The model under review builds one solid part; all positions refer to its coordinate system, in mm. Face numbers are marked on the shaded views. A direction names the side the tool comes from. Round coordinates to 2 decimals unless told otherwise and drop trailing zeros. Write each loop counter-clockwise with the first axis right and the second up, starting at its lowest first coordinate (ties: lowest second). Pieces come first, ordered by that corner, then holes. Notation, with made-up numbers: (54.5, 28) - (65.5, 28) arc R16 ccw to (65.5, 37) - close; hole circle Ø5 at (27.25, 4.5). An arc over 180 degrees is marked (long way). Use one line per item in the form item = value.
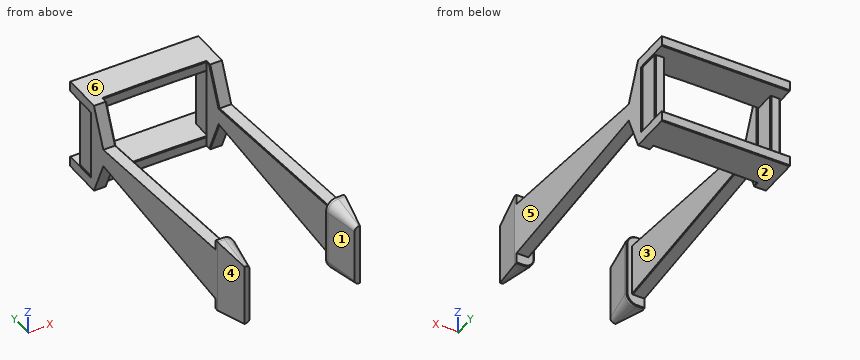
from build123d import *

# Parameters (mm, degrees)
BOSS_EXTRUDE1_DEPTH           = 30
SKETCH2_W                     = 26.926999998
SKETCH2_H                     = 60
BOSS_EXTRUDE2_DEPTH           = 200
BOSS_EXTRUDE3_START           = 30
BOSS_EXTRUDE3_DEPTH           = 30
BOSS_EXTRUDE4_DEPTH           = 4.0365
BOSS_EXTRUDE4_DEPTH_BACK      = 30.9635
BOSS_EXTRUDE5_DEPTH           = 10
FILLET1_R                     = 30
SKETCH7_W                     = 260
SKETCH7_H                     = 710
CUT_EXTRUDE1_DEPTH            = 768.843643003
CHAMFER1_SIZE                 = 2
CHAMFER2_SIZE                 = 2
CHAMFER3_SIZE                 = 2
CHAMFER4_SIZE                 = 2
CHAMFER6_SIZE                 = 2
BOSS_EXTRUDE6_DEPTH           = 99
BOSS_EXTRUDE6_DRAFT           = 10
BOSS_EXTRUDE6_PROFILE_2_DEPTH = 99
BOSS_EXTRUDE6_PROFILE_2_DRAFT = 10


with BuildPart() as part:
    # Sketch1 → Boss-Extrude1 (new body)
    with BuildSketch(Plane.XY):
        with BuildLine():
            Line((0, 0), (361.02, 0))
            Line((361.02, 0), (361.02, -100))
            Line((361.02, -100), (326.02, -100))
            ThreePointArc((326.02, -100), (180.51, -98.235310481), (35, -100))
            Line((35, -100), (0, -100))
            Line((0, -100), (0, 0))
        make_face()
    extrude(amount=BOSS_EXTRUDE1_DEPTH)

    # Sketch2 → Boss-Extrude2 (add)
    with BuildSketch(Plane(origin=(0, 0, 0), x_dir=(-1, 0, 0), z_dir=(0, 0, -1))):
        with Locations((-343.52, -70)):
            Rectangle(SKETCH2_W, SKETCH2_H)
        with Locations((-17.5, -70)):
            Rectangle(SKETCH2_W, SKETCH2_H)
    extrude(amount=BOSS_EXTRUDE2_DEPTH)

    # Sketch3 → Boss-Extrude3 (add)
    with BuildSketch(Plane(origin=(0, 0, -200), x_dir=(-1, 0, 0), z_dir=(0, 0, -1)).offset(BOSS_EXTRUDE3_START)):
        with BuildLine():
            Line((0, -100), (0, 0))
            Line((0, 0), (-361.02, 0))
            Line((-361.02, 0), (-361.02, -100))
            Line((-361.02, -100), (-326.02, -100))
            ThreePointArc((-326.02, -100), (-180.51, -98.235310481), (-35, -100))
            Line((-35, -100), (0, -100))
        make_face()
    extrude(amount=-BOSS_EXTRUDE3_DEPTH)

    # Sketch5 → Boss-Extrude4 (add, two sides: drawn at the far end of the back side and taken through both)
    with BuildSketch(Plane.ZY.offset(-4.036500001).offset(-BOSS_EXTRUDE4_DEPTH_BACK)):
        Polygon((-200, -100), (0, -100), (30, -100), (30, -115), (-75, -160), (-25, -700), (-100, -700), (-175, -700), (-125, -160), (-230, -115), (-230, -100), align=None)
    extrude(amount=BOSS_EXTRUDE4_DEPTH + BOSS_EXTRUDE4_DEPTH_BACK)

    # Sketch6 → Boss-Extrude5 (add)
    with BuildSketch(Plane.XZ.offset(700)):
        Polygon((0, -25), (0, 5), (50, 5), (50, -205), (0, -205), (0, -175), align=None)
    extrude(amount=BOSS_EXTRUDE5_DEPTH)

    # Fillet1
    fillet1_edges = [part.edges().sort_by_distance(p)[0] for p in [
        (50, -705, -205),
        (50, -705, 5),
    ]]
    fillet(fillet1_edges, radius=FILLET1_R)

    # Sketch7 → Cut-Extrude1 (cut, through all)
    with BuildSketch(Plane(origin=(180.51, 0, 0), x_dir=(0, 0, -1), z_dir=(1, 0, 0))):
        with Locations((100, -355)):
            Rectangle(SKETCH7_W, SKETCH7_H)
    extrude(amount=CUT_EXTRUDE1_DEPTH, mode=Mode.SUBTRACT)

    # Mirror2: part across plane


with BuildPart() as part_1:
    add(part.part)
    add(part.part.mirror(Plane(origin=(180.51, 0, 0), x_dir=(0, 0, 1), z_dir=(1, 0, 0))))

    # Chamfer1
    chamfer1_edges = [part_1.edges().sort_by_distance(p)[0] for p in [
        (180.51, 0, 30),
        (180.51, 0, 0),
        (180.51, 0, -200),
        (180.51, 0, -230),
    ]]
    chamfer(chamfer1_edges, length=CHAMFER1_SIZE)

    # Chamfer2
    chamfer2_edges = [part_1.edges().sort_by_distance(p)[0] for p in [
        (356.983499999, -40, -100),
        (330.056500001, -40, -100),
        (4.036500001, -40, -100),
        (30.963499999, -40, -100),
    ]]
    chamfer(chamfer2_edges, length=CHAMFER2_SIZE)

    # Chamfer3
    chamfer3_edges = [part_1.edges().sort_by_distance(p)[0] for p in [
        (326.019999999, -107.5, -230),
        (326.019999999, -137.5, -177.5),
        (326.019999999, -430, -150),
        (326.019999999, -430, -50),
        (326.019999999, -137.5, -22.5),
        (326.019999999, -107.5, 30),
        (35.000000001, -107.5, 30),
        (35.000000001, -137.5, -22.5),
        (35.000000001, -430, -50),
        (35.000000001, -430, -150),
        (35.000000001, -137.5, -177.5),
        (35.000000001, -107.5, -230),
    ]]
    chamfer(chamfer3_edges, length=CHAMFER3_SIZE)

    # Chamfer4
    chamfer4_edges = [part_1.edges().sort_by_distance(p)[0] for p in [
        (50, -700, -100),
        (10, -700, 5),
        (41.213203436, -700, -3.786796564),
        (41.213203436, -700, -196.213203436),
        (311.02, -700, -100),
        (351.02, -700, 5),
        (351.02, -700, -205),
        (319.806796564, -700, -196.213203436),
        (319.806796564, -700, -3.786796564),
        (10, -700, -205),
    ]]
    chamfer(chamfer4_edges, length=CHAMFER4_SIZE)

    # Chamfer6
    # the kernel refuses this chamfer: 2 mm, written as the material it takes off along each edge
    with BuildSketch(Plane(origin=(180.51, -6098.235310479, 30), x_dir=(0.025441959758898923, 0.9996763009512762, 0), z_dir=(0.9996763009512762, -0.025441959758898923, 0))) as chamfer6_piece_1_section:
        Polygon((5999.999999998 + CHAMFER6_SIZE, 0), (5999.999999998, -CHAMFER6_SIZE), (5999.999999998, 0), align=None)
    chamfer6_piece_1 = revolve(axis=Axis((180.51, -6098.235310479, 30), (0, 0, 1)), revolution_arc=2.915748449, mode=Mode.PRIVATE)
    chamfer6_piece_1 = split(chamfer6_piece_1, bisect_by=Plane(origin=(327.145000629, -99.268037673, 29.12500063), z_dir=(-0.7071067811865476, 0, 0.7071067811865476)), keep=Keep.TOP, mode=Mode.PRIVATE)
    chamfer6_piece_1 = split(chamfer6_piece_1, bisect_by=Plane(origin=(180.135000332, -99.268037673, -117.135000331), z_dir=(0.7071067811865476, 0, 0.7071067811865476)), keep=Keep.TOP, mode=Mode.PRIVATE)
    add(chamfer6_piece_1, mode=Mode.SUBTRACT)
    with BuildSketch(Plane(origin=(180.51, -6098.235310479, 0), x_dir=(0.02510863351858876, 0.9996847285633752, 0), z_dir=(0.9996847285633752, -0.02510863351858876, 0))) as chamfer6_piece_2_section:
        Polygon((5999.999999998 + CHAMFER6_SIZE, 0), (5999.999999998, CHAMFER6_SIZE), (5999.999999998, 0), align=None)
    chamfer6_piece_2 = revolve(axis=Axis((180.51, -6098.235310479, 0), (0, 0, 1)), revolution_arc=2.877539868, mode=Mode.PRIVATE)
    chamfer6_piece_2 = split(chamfer6_piece_2, bisect_by=Plane(origin=(328.004034253, -100, 0.650481022), z_dir=(0, 1, 0)), keep=Keep.TOP, mode=Mode.PRIVATE)
    chamfer6_piece_2 = split(chamfer6_piece_2, bisect_by=Plane(origin=(330.056500001, -99.349322449, 0.650481022), z_dir=(-1, 0, 0)), keep=Keep.TOP, mode=Mode.PRIVATE)
    chamfer6_piece_2 = split(chamfer6_piece_2, bisect_by=Plane(origin=(30.963499999, -99.349322449, 0.650481022), z_dir=(1, 0, 0)), keep=Keep.TOP, mode=Mode.PRIVATE)
    add(chamfer6_piece_2, mode=Mode.SUBTRACT)
    with BuildSketch(Plane(origin=(180.51, -6098.235310479, -200), x_dir=(-0.025108633518586027, 0.9996847285633753, 0), z_dir=(-0.9996847285633753, -0.025108633518586027, 0))) as chamfer6_piece_3_section:
        Polygon((5999.999999998 + CHAMFER6_SIZE, 0), (5999.999999998, CHAMFER6_SIZE), (5999.999999998, 0), align=None)
    chamfer6_piece_3 = revolve(axis=Axis((180.51, -6098.235310479, -200), (0, 0, -1)), revolution_arc=2.877539868, mode=Mode.PRIVATE)
    chamfer6_piece_3 = split(chamfer6_piece_3, bisect_by=Plane(origin=(33.015965747, -100, -200.650481022), z_dir=(0, 1, 0)), keep=Keep.TOP, mode=Mode.PRIVATE)
    chamfer6_piece_3 = split(chamfer6_piece_3, bisect_by=Plane(origin=(330.056500001, -99.349322449, -200.650481022), z_dir=(-1, 0, 0)), keep=Keep.TOP, mode=Mode.PRIVATE)
    chamfer6_piece_3 = split(chamfer6_piece_3, bisect_by=Plane(origin=(30.963499999, -99.349322449, -200.650481022), z_dir=(1, 0, 0)), keep=Keep.TOP, mode=Mode.PRIVATE)
    add(chamfer6_piece_3, mode=Mode.SUBTRACT)
    with BuildSketch(Plane(origin=(180.51, -6098.235310479, -230), x_dir=(-0.025441959758894937, 0.9996763009512762, 0), z_dir=(-0.9996763009512762, -0.025441959758894937, 0))) as chamfer6_piece_4_section:
        Polygon((5999.999999998 + CHAMFER6_SIZE, 0), (5999.999999998, -CHAMFER6_SIZE), (5999.999999998, 0), align=None)
    chamfer6_piece_4 = revolve(axis=Axis((180.51, -6098.235310479, -230), (0, 0, -1)), revolution_arc=2.915748449, mode=Mode.PRIVATE)
    chamfer6_piece_4 = split(chamfer6_piece_4, bisect_by=Plane(origin=(180.884999668, -99.268037673, -82.864999669), z_dir=(-0.7071067811865476, 0, -0.7071067811865476)), keep=Keep.TOP, mode=Mode.PRIVATE)
    chamfer6_piece_4 = split(chamfer6_piece_4, bisect_by=Plane(origin=(33.874999371, -99.268037673, -229.12500063), z_dir=(0.7071067811865476, 0, -0.7071067811865476)), keep=Keep.TOP, mode=Mode.PRIVATE)
    add(chamfer6_piece_4, mode=Mode.SUBTRACT)


with BuildPart() as boss_extrude6_tool:
    # Sketch10 → Boss-Extrude6 (with draft: the straight prism first)
    with BuildSketch(Plane.XZ.offset(710)):
        with BuildLine():
            Line((341.02, -205), (361.02, -205))
            Line((361.02, -205), (361.02, 5))
            Line((361.02, 5), (341.02, 5))
            ThreePointArc((341.02, 5), (319.806796564, -3.786796564), (311.02, -25))
            Line((311.02, -25), (311.02, -175))
            ThreePointArc((311.02, -175), (319.806796564, -196.213203436), (341.02, -205))
        make_face()
    extrude(amount=BOSS_EXTRUDE6_DEPTH)
    # Boss-Extrude6: the draft: its side faces are tilted about the plane it starts from
    boss_extrude6_sides = [boss_extrude6_tool.faces().sort_by_distance(p)[0] for p in [
        (351.02, -759.5, -205),
        (361.02, -759.5, -100),
        (351.02, -759.5, 5),
        (319.806796564, -759.5, -3.786796564),
        (311.02, -759.5, -100),
        (319.806796564, -759.5, -196.213203436),
    ]]
    draft(boss_extrude6_sides, Plane.XZ.offset(710), BOSS_EXTRUDE6_DRAFT)


with BuildPart() as part_2:
    add(part_1.part)

    # Boss-Extrude6: add boss_extrude6_tool
    add(boss_extrude6_tool.part)


with BuildPart() as boss_extrude6_profile_2_tool:
    # Sketch10 → Boss-Extrude6 profile 2 (with draft: the straight prism first)
    with BuildSketch(Plane.XZ.offset(710)):
        with BuildLine():
            Line((0, -205), (20, -205))
            ThreePointArc((20, -205), (41.213203436, -196.213203436), (50, -175))
            Line((50, -175), (50, -25))
            ThreePointArc((50, -25), (41.213203436, -3.786796564), (20, 5))
            Line((20, 5), (0, 5))
            Line((0, 5), (0, -205))
        make_face()
    extrude(amount=BOSS_EXTRUDE6_PROFILE_2_DEPTH)
    # Boss-Extrude6 profile 2: the draft: its side faces are tilted about the plane it starts from
    boss_extrude6_profile_2_sides = [boss_extrude6_profile_2_tool.faces().sort_by_distance(p)[0] for p in [
        (10, -759.5, -205),
        (41.213203436, -759.5, -196.213203436),
        (50, -759.5, -100),
        (41.213203436, -759.5, -3.786796564),
        (10, -759.5, 5),
        (0, -759.5, -100),
    ]]
    draft(boss_extrude6_profile_2_sides, Plane.XZ.offset(710), BOSS_EXTRUDE6_PROFILE_2_DRAFT)


with BuildPart() as part_3:
    add(part_2.part)

    # Boss-Extrude6 profile 2: add boss_extrude6_profile_2_tool
    add(boss_extrude6_profile_2_tool.part)


solid = part_3.part
(1) Add section B-B on y = -403.5. Write out the cut boundary in (x, z).
Geometry results:
outline = (0, -147.55) - (33, -147.55) - (35, -145.54) - (35, -54.46) - (33, -52.45) - (0, -52.45) - close; (326.02, -145.54) - (328.02, -147.55) - (361.02, -147.55) - (361.02, -52.45) - (328.02, -52.45) - (326.02, -54.46) - close
(2) To check wall thickness, follow L1, parallel to Z at x = 248, y = -84.5; L2, parallel to X at y = -120.5, z = -45; L3, parallel to X at y = -57, z = -125.5. State the ranges of each line that lie inside material, in increasing order.
Geometry results:
L1 = -230 to -200, 0 to 30
L2 = 0 to 35, 326.02 to 361.02
L3 = 4.04 to 30.96, 330.06 to 356.98
(3) The part is to be moulded in two halves that separate along X. For the marked faces 3, 4, 5 and 6, say which applies: +X half, -X half, draft (parallel to the pull), parting line (faces both ways), or undercut.
Geometry results:
face_3 = undercut
face_4 = -X half
face_5 = +X half
face_6 = draft
(4) Add section C-C on z = -38.5. Count the separate pieces of the cut face and the enclosed holes in it, then the cut area to 3 significant figures.
Geometry results:
separate_pieces = 4
enclosed_holes = 0
area = 23,900 mm2
(5) Add section D-D on y = -234.5. Write out the cut boundary in (x, z), then the cut area to 3 significant figures.
Geometry results:
outline = (0, -131.9) - (33, -131.9) - (35, -129.89) - (35, -70.11) - (33, -68.1) - (0, -68.1) - close; (326.02, -129.89) - (328.02, -131.9) - (361.02, -131.9) - (361.02, -68.1) - (328.02, -68.1) - (326.02, -70.11) - close
area = 4,460 mm2
(6) Machinability: for the marked faces 1 and 2, which of the approach directions +Z, -Z, +X, -X, +Y, -Y give a long, thin tool a straight path to every point of the face, cutting with its end or side? Answer none if there is none.
Geometry results:
face_1 = +Z, -Z, -Y
face_2 = -Z, +X, -X, +Y, -Y
(7) Insertion check: P1, Ø6.5, axis at x = 346.5, y = -704.5, coming from the +Z side; P2, Ø17.5, axis at y = -58.5, z = -127.5, coming from the +X side; P3, Ø2, axis at x = 2, z = -63.5, coming from the +Y side. Each pin has a flat end and moves straight along its axis. Give the tip position at first contact, or say it passes through.
Geometry results:
P1 = 5
P2 = 356.98
P3 = -100
